```python
from build123d import *

# Parameters (mm, degrees)
SKETCH1_R           = 2.6289
SKETCH1_R_2         = 2.0193
SKETCH1_R_3         = 12.7
BOSS_EXTRUDE1_DEPTH = 6.35
SKETCH8_R           = 3.2639
CUT_EXTRUDE1_DEPTH  = 7.35
CUT_EXTRUDE2_START  = -2.38125
SKETCH9_R           = 3.175
CUT_EXTRUDE2_DEPTH  = 12.41425
CIRPATTERN1_COUNT   = 4
CIRPATTERN1_ANGLE   = 33
SKETCH10_R          = 3.2639
CUT_EXTRUDE3_DEPTH  = 7.35


with BuildPart() as part:
    # Sketch1 → Boss-Extrude1 (new body)
    with BuildSketch(Plane(origin=(0, 0, 0), x_dir=(0, 0, -1), z_dir=(1, 0, 0))):
        with BuildLine():
            ThreePointArc((136.202701987, 114.287637002), (167.077347976, 60.811181483), (177.8, 0))
            Line((177.8, 0), (177.8, -50.8))
            Line((177.8, -50.8), (228.6, -50.8))
            Line((228.6, -50.8), (228.6, -15.875))
            Line((228.6, -15.875), (276.225, 0))
            ThreePointArc((276.225, 0), (270.787208867, 54.539326538), (254.687933194, 106.93132053))
            Line((254.687933194, 106.93132053), (250.70144255, 121.427783901))
            Line((250.70144255, 121.427783901), (237.590987118, 143.182690436))
            Line((237.590987118, 143.182690436), (224.480531685, 164.937596971))
            Line((224.480531685, 164.937596971), (197.194423369, 161.00537172))
            Line((197.194423369, 161.00537172), (166.921891726, 156.642770358))
            Line((166.921891726, 156.642770358), (142.599980657, 136.23426375))
            Line((142.599980657, 136.23426375), (136.202701987, 114.287637002))
        make_face()
        with Locations((190.5, -38.1)):
            Circle(SKETCH1_R, mode=Mode.SUBTRACT)
        with Locations((215.9, -38.1)):
            Circle(SKETCH1_R, mode=Mode.SUBTRACT)
        with BuildLine():
            Line((210.919197755, 88.15357065), (219.558563098, 92.182172871))
            ThreePointArc((219.558563098, 92.182172871), (233.437249023, 47.016660809), (238.125, 0))
            Line((238.125, 0), (228.6, 0))
            ThreePointArc((228.6, 0), (224.136218188, 44.954595945), (210.919197755, 88.15357065))
        make_face(mode=Mode.SUBTRACT)
        with Locations((191.182546707, 136.184784997)):
            Circle(SKETCH1_R_2, mode=Mode.SUBTRACT)
        with Locations((209.723530589, 105.418701127)):
            Circle(SKETCH1_R_2, mode=Mode.SUBTRACT)
        with Locations((215.836080583, 130.072235003)):
            Circle(SKETCH1_R_3, mode=Mode.SUBTRACT)
        with Locations((240.489614459, 123.959685009)):
            Circle(SKETCH1_R_2, mode=Mode.SUBTRACT)
        with Locations((221.948630577, 154.725768879)):
            Circle(SKETCH1_R_2, mode=Mode.SUBTRACT)
    extrude(amount=BOSS_EXTRUDE1_DEPTH)

    # Sketch8 → Cut-Extrude1 (cut, through all)
    with BuildSketch(Plane.ZY):
        with Locations((-218.241353484, 19.093644342)):
            Circle(SKETCH8_R)
        with Locations((-192.938008153, 16.879888477)):
            Circle(SKETCH8_R)
        with Locations((-210.588406038, 60.385253726)):
            Circle(SKETCH8_R)
        with Locations((-186.172358961, 53.384064888)):
            Circle(SKETCH8_R)
        with Locations((-195.197254287, 99.45796873)):
            Circle(SKETCH8_R)
        with Locations((-172.565688572, 87.926610037)):
            Circle(SKETCH8_R)
        with Locations((-172.633455846, 134.876037707)):
            Circle(SKETCH8_R)
        with Locations((-152.617982705, 119.238236234)):
            Circle(SKETCH8_R)
        with BuildLine():
            Line((-201.035193399, 27.787109942), (-202.806198092, 7.544433676))
            ThreePointArc((-202.806198092, 7.544433676), (-206.933763272, 4.080995257), (-210.397201691, 8.208560436))
            Line((-210.397201691, 8.208560436), (-208.626196999, 28.451236701))
            ThreePointArc((-208.626196999, 28.451236701), (-204.498631819, 31.914675121), (-201.035193399, 27.787109942))
        make_face()
        with BuildLine():
            Line((-192.039580138, 65.635905756), (-197.640531208, 46.103068095))
            ThreePointArc((-197.640531208, 46.103068095), (-202.353116595, 43.490839359), (-204.965345331, 48.203424746))
            Line((-204.965345331, 48.203424746), (-199.364394261, 67.736262407))
            ThreePointArc((-199.364394261, 67.736262407), (-194.651808874, 70.348491143), (-192.039580138, 65.635905756))
        make_face()
        with BuildLine():
            Line((-182.776820638, 104.532276267), (-192.001907592, 86.427023695))
            ThreePointArc((-192.001907592, 86.427023695), (-190.336876539, 81.302585034), (-185.212437878, 82.967616087))
            Line((-185.212437878, 82.967616087), (-175.987350923, 101.072868659))
            ThreePointArc((-175.987350923, 101.072868659), (-177.652381977, 106.19730732), (-182.776820638, 104.532276267))
        make_face()
        with BuildLine():
            Line((-159.472997023, 137.487185455), (-171.983238202, 121.474806942))
            ThreePointArc((-171.983238202, 121.474806942), (-171.326587452, 116.12681575), (-165.978596259, 116.7834665))
            Line((-165.978596259, 116.7834665), (-153.468355081, 132.795845013))
            ThreePointArc((-153.468355081, 132.795845013), (-154.125005831, 138.143836206), (-159.472997023, 137.487185455))
        make_face()
    extrude(amount=-CUT_EXTRUDE1_DEPTH, mode=Mode.SUBTRACT)

    # Sketch9 → Cut-Extrude2 (cut)
    with BuildSketch(Plane(origin=(0, 18.329898569, -209.511699345), x_dir=(0, -0.087155743, 0.996194698), z_dir=(-1, 0, 0)).offset(CUT_EXTRUDE2_START)):
        Circle(SKETCH9_R)
        with Locations((7.62, 0)):
            Circle(SKETCH9_R)
    cut_extrude2 = extrude(amount=CUT_EXTRUDE2_DEPTH, mode=Mode.SUBTRACT)

    # CirPattern1: Cut-Extrude2 ×4 about axis
    cirpattern1_axis = Axis((0, 0, 0), (1, 0, 0))
    for i in range(1, CIRPATTERN1_COUNT):
        add(cut_extrude2.rotate(cirpattern1_axis, i * CIRPATTERN1_ANGLE / (CIRPATTERN1_COUNT - 1)), mode=Mode.SUBTRACT)

    # Sketch10 → Cut-Extrude3 (cut, through all)
    with BuildSketch(Plane.ZY):
        with Locations((-188.512295871, 152.654247257)):
            Circle(SKETCH10_R)
    extrude(amount=-CUT_EXTRUDE3_DEPTH, mode=Mode.SUBTRACT)


solid = part.part
```
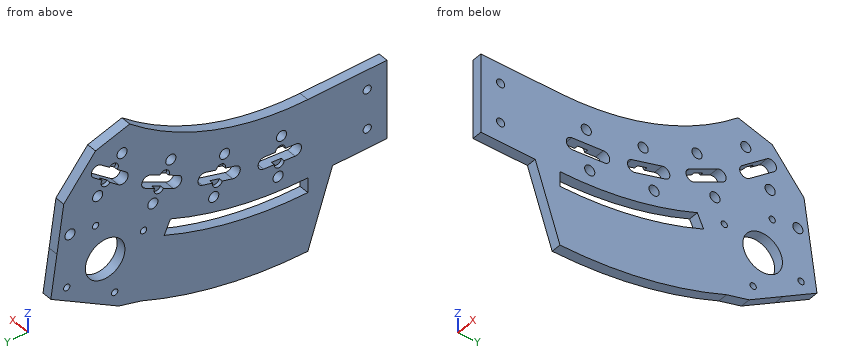
Can you work these out from the model? Positions are in its coordinate system, mm. Give positions to 0.01 mm unless a question says otherwise; leave off trailing zeros. Loops run counter-clockwise (first coordinate to the right, second up) from the corner with the lowest first, then second, coordinate; pieces in that order, holes last. Notation, with made-up numbers: M 55,-13 L 110,-13 A17 ccw 110,19 Z; hole C 82.5,11.25 d3. An arc over 180 degrees is marked long. One line per item, written item: value.
(1) Suppose I cut it at C-C on z = -266.5. List the corners of the cut face in (x, y) for me.
Returned:
outline: M 0,-3.24 L 6.35,-3.24 L 6.35,72.65 L 0,72.65 Z
(2) Suppose I cut it at D-D on y = -5. List the corners of the cut face in (x, z) for me (3 decimals).
Returned:
outline: M 0,-261.225 L 6.35,-261.225 L 6.35,-177.8 L 0,-177.8 Z
(3) Will these pins go through, and if not, where does the flat tip stop? pin 1 (1.2 mm diameter, centred on y = 57.5, z = -193, fed in from -X); pin 2 (1.9 mm diameter, centred on x = 3.5, y = -39, fed in from -Z); pin 3 (1 mm diameter, centred on x = 5, z = -158.5, fed in from -Y).
Returned:
pin 1: x = 2.38
pin 2: z = -228.6
pin 3: y = 79.57
(4) Suppose I cut it at B-B on x = 1.25. Count the separate pieces of the cut face and the enclosed holes in it, plus the area to 3 significant figures.
Returned:
separate pieces: 1
enclosed holes: 21
area: 16,400 mm^2
(5) I need wall thicknesses on line 1 (Y direction, x = 1.25, z = -195); line 2 (Z direction, x = 1.25, y = 57); line 3 (Z direction, x = 3, y = 21). Which ranges of each line are inside material? Lowest first, please.
Returned:
line 1: -50.8 to 14.35, 19.41 to 52.7, 70.43 to 96.2, 102.72 to 160.69
line 2: -270.28 to -231.2, -221.38 to -205.19, -191.87 to -168.42
line 3: -275.43 to -237.2, -227.63 to -220.89, -215.59 to -209.28, -201.63 to -176.56
(6) Suppose I cut it at A-A on y = 36.5. List the corners of the cut face in (x, z) for me, plus the area to 3 significant figures.
Returned:
outline: M 0,-273.8 L 6.35,-273.8 L 6.35,-235.31 L 0,-235.31 Z; M 0,-225.67 L 6.35,-225.67 L 6.35,-174.01 L 0,-174.01 Z
area: 572 mm^2
